from build123d import *

# Parameters (mm, degrees)
CYLINDER_R       = 0.6
CYLINDER_DEPTH   = 10
ARRAY001_X_COUNT = 2
ARRAY001_X_PITCH = 15
BOX007_W         = 18.6
BOX007_H         = 45
BOX007_DEPTH     = 1.6
BOX006_W         = 17.2
BOX006_H         = 45.1
BOX006_DEPTH     = 6.1
BOX_W            = 21.6
BOX_H            = 46.5
BOX_DEPTH        = 7.6
FILLET_R         = 1
BOX008_W         = 3
BOX008_H         = 3
BOX008_DEPTH     = 4.5
ARRAY_X_COUNT    = 2
ARRAY_X_PITCH    = 15


with BuildPart() as hole_array001:
    # Cylinder → Cylinder (new body)
    with BuildSketch(Plane.XY):
        Circle(CYLINDER_R)
    extrude(amount=CYLINDER_DEPTH)

    # Array001 X: hole array001 ×2


with BuildPart() as hole_array001_1:
    add(hole_array001.part)
    with Locations(*[(i * ARRAY001_X_PITCH, 0, 0) for i in range(1, ARRAY001_X_COUNT)]):
        add(hole_array001.part)


with BuildPart() as hole_array001_2:
    # Array001 placement: moved
    add(hole_array001_1.part.moved(Location((3.3, 4, 0))))


with BuildPart() as pcb_extract_cube:
    # Box007 → Box007 (new body)
    with BuildSketch(Plane(origin=(1.5, 1.5, 4.5), x_dir=(1, 0, 0), z_dir=(0, 0, 1))):
        with Locations((9.3, 22.5)):
            Rectangle(BOX007_W, BOX007_H)
    extrude(amount=BOX007_DEPTH)


with BuildPart() as extract_fusion:
    # Box006 → Box006 (new body)
    with BuildSketch(Plane(origin=(2.2, 2.2, 1.5), x_dir=(1, 0, 0), z_dir=(0, 0, 1))):
        with Locations((8.6, 22.55)):
            Rectangle(BOX006_W, BOX006_H)
    extrude(amount=BOX006_DEPTH)

    # Fusion: union pcb extract cube
    add(pcb_extract_cube.part)


with BuildPart() as body_cut004:
    # Box → Box (new body)
    with BuildSketch(Plane.XY):
        with Locations((10.8, 23.25)):
            Rectangle(BOX_W, BOX_H)
    extrude(amount=BOX_DEPTH)

    # Fillet
    fillet_edges = [body_cut004.edges().sort_by_distance(p)[0] for p in [
        (0, 0, 3.8),
        (0, 46.5, 3.8),
        (21.6, 0, 3.8),
        (21.6, 46.5, 3.8),
    ]]
    fillet(fillet_edges, radius=FILLET_R)

    # Cut003007: cut extract fusion
    add(extract_fusion.part, mode=Mode.SUBTRACT)


with BuildPart() as body_cut005:
    # Box008 → Box008 (new body)
    with BuildSketch(Plane(origin=(-1.5, -1.5, 0), x_dir=(1, 0, 0), z_dir=(0, 0, 1))):
        with Locations((1.5, 1.5)):
            Rectangle(BOX008_W, BOX008_H)
    extrude(amount=BOX008_DEPTH)

    # Array X: body cut005 ×2


with BuildPart() as body_cut005_1:
    add(body_cut005.part)
    with Locations(*[(i * ARRAY_X_PITCH, 0, 0) for i in range(1, ARRAY_X_COUNT)]):
        add(body_cut005.part)


with BuildPart() as body_cut005_2:
    # Array placement: moved
    add(body_cut005_1.part.moved(Location((3.3, 4, 0))))

    # Fusion006: union body cut004
    add(body_cut004.part)

    # Cut003008: cut hole array001
    add(hole_array001_2.part, mode=Mode.SUBTRACT)


solid = body_cut005_2.part
Geometry check sheet. Reference: the model listing, model coordinates, mm. A direction names the side the tool comes from. Give positions to 0.01 mm unless a question says otherwise; leave off trailing zeros. Loops run counter-clockwise (first coordinate to the right, second up) from the corner with the lowest first, then second, coordinate; pieces in that order, holes last. Notation, with made-up numbers: M 6,-15.5 L 20,-15.5 A25 ccw 20,10.5 Z; hole C 24,23.5 d8. An arc over 180 degrees is marked long. Answer as a JSON object with one key per item and string values. Group by question number.
Item 1: Access from +Z, -Z, +X, -X, +Y, -Y to the whole of each face (thin tool, end or side, straight path). Record for faces 1 (the flat face through (1.5, 24, 5)), 2 (the flat face through (4.8, 4, 3)), 3 (the flat face through (11, 46.5, 1)), 4 (the flat face through (18, 2.5, 3)).
Item 2: Sectioned sample at D-D on z = 6.75. Record the boundary of the cut face in (x, y).
Item 3: Sectioned sample at B-B on z = 3.25. Record the boundary of the cut face in (x, y), plus the area to 3 significant figures.
Item 4: Sectioned sample at A-A on x = 3.3. Record the boundary of the cut face in (y, z).
Item 5: Sectioned sample at C-C on y = 4. Record the boundary of the cut face in (x, z), plus the area to 3 significant figures.
Item 6: Material ranges on L1, parallel to Y at x = 3.3, z = 3.45; L2, parallel to X at y = 4, z = 2.35; L3, parallel to X at y = 4, z = 1.4, recorded low to high.
Item 7: Mould release check, pull along Y, two halves, no side actions. Record for faces 5 (the cylindrical face through (18.854, 3.77, 2.218)), 6 (the flat face through (11, 0, 4)), 7 (the flat face through (3, 2.5, 3)), 8 (the flat face through (3, 5.5, 3)): pulls with the +Y half, pulls with the -Y half, needs draft (parallel to the pull), parting line crosses it, or undercut.
Item 8: Gauge pin test, flat ends, axial feed: pin 1 (1.2 mm diameter, centred on x = 9, z = 7, fed in from +Y); pin 2 (1 mm diameter, centred on x = 3.3, y = 4, fed in from +Z); pin 3 (10 mm diameter, centred on x = 5, y = 9.5, fed in from +Z); pin 4 (2 mm diameter, centred on x = 7, y = 12, fed in from +Z). Record the tip position at first contact, or that the pin passes through.
Findings below:
{
 "1": {"face 1": "+Y", "face 2": "+Z, +Y", "face 3": "+Z, -Z, +X, -X, +Y", "face 4": "+Z"},
 "2": {"outline": "M 0,1 A1 ccw 1,0 L 20.6,0 A1 ccw 21.6,1 L 21.6,45.5 A1 ccw 20.6,46.5 L 19.4,46.5 L 19.4,2.2 L 2.2,2.2 L 2.2,46.5 L 1,46.5 A1 ccw 0,45.5 Z"},
 "3": {"outline": "M 0,1 A1 ccw 1,0 L 20.6,0 A1 ccw 21.6,1 L 21.6,45.5 A1 ccw 20.6,46.5 L 19.4,46.5 L 19.4,5.5 L 16.8,5.5 L 16.8,2.5 L 19.4,2.5 L 19.4,2.2 L 2.2,2.2 L 2.2,2.5 L 4.8,2.5 L 4.8,5.5 L 2.2,5.5 L 2.2,46.5 L 1,46.5 A1 ccw 0,45.5 Z; hole C 3.3,4 d1.2; hole C 18.3,4 d1.2", "area": "255 mm2"},
 "4": {"outline": "M 0,0 L 3.4,0 L 3.4,4.5 L 2.5,4.5 L 2.5,1.5 L 2.2,1.5 L 2.2,4.5 L 1.5,4.5 L 1.5,6.1 L 2.2,6.1 L 2.2,7.6 L 0,7.6 Z; M 4.6,0 L 46.5,0 L 46.5,1.5 L 5.5,1.5 L 5.5,4.5 L 4.6,4.5 Z"},
 "5": {"outline": "M 0,0 L 2.7,0 L 2.7,4.5 L 1.5,4.5 L 1.5,6.1 L 2.2,6.1 L 2.2,7.6 L 0,7.6 Z; M 3.9,0 L 17.7,0 L 17.7,4.5 L 16.8,4.5 L 16.8,1.5 L 4.8,1.5 L 4.8,4.5 L 3.9,4.5 Z; M 18.9,0 L 21.6,0 L 21.6,7.6 L 19.4,7.6 L 19.4,6.1 L 20.1,6.1 L 20.1,4.5 L 18.9,4.5 Z", "area": "61.8 mm2"},
 "6": {"L1": "0 to 2.2, 2.5 to 3.4, 4.6 to 5.5", "L2": "0 to 2.7, 3.9 to 4.8, 16.8 to 17.7, 18.9 to 21.6", "L3": "0 to 2.7, 3.9 to 17.7, 18.9 to 21.6"},
 "7": {"face 5": "undercut", "face 6": "pulls with the -Y half", "face 7": "undercut", "face 8": "pulls with the +Y half"},
 "8": {"pin 1": "y = 2.2", "pin 2": "through", "pin 3": "z = 7.6", "pin 4": "z = 1.5"}
}
